Build history of the part. All positions in model axes, mm. Round coordinates to 2 decimals unless told otherwise and drop trailing zeros. Write each loop counter-clockwise with the first axis right and the second up, starting at its lowest first coordinate (ties: lowest second). Pieces come first, ordered by that corner, then holes. Notation, with made-up numbers: (24.25, 55.5) - (56.25, 55.5) arc R12 cw to (56.25, 72.5) - close; hole circle Ø2 at (12.5, 62). An arc over 180 degrees is marked (long way). Write each question's results on one line, items separated by ' | '.
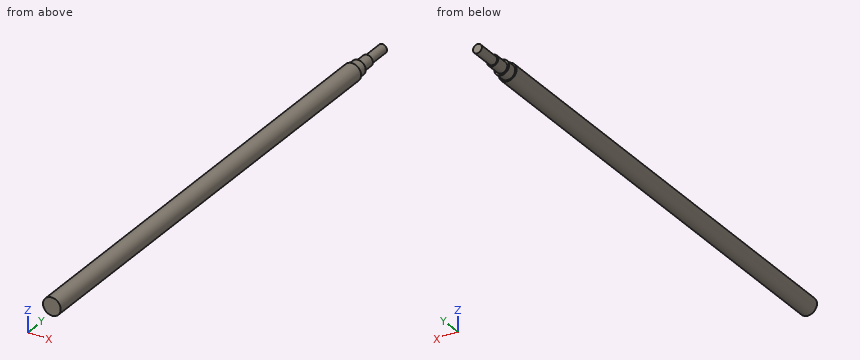
from build123d import *

# Parameters (mm, degrees)
SKETCH1_R           = 9.525
BOSS_EXTRUDE1_DEPTH = 500
SKETCH2_R           = 8
BOSS_EXTRUDE2_DEPTH = 10
SKETCH3_R           = 6
BOSS_EXTRUDE3_DEPTH = 15
SKETCH4_R           = 4.7625
BOSS_EXTRUDE4_DEPTH = 25.4


with BuildPart() as part:
    # Sketch1 → Boss-Extrude1 (new body)
    with BuildSketch(Plane(origin=(0, 0, 0), x_dir=(1, 0, 0), z_dir=(0, 1, 0))):
        with Locations(Location((0, 0, 0), (0, 0, 270))):
            Circle(SKETCH1_R)
    extrude(amount=BOSS_EXTRUDE1_DEPTH)

    # Sketch2 → Boss-Extrude2 (add)
    with BuildSketch(Plane(origin=(0, 500, 0), x_dir=(1, 0, 0), z_dir=(0, 1, 0))):
        with Locations(Location((0, 0, 0), (0, 0, 270))):
            Circle(SKETCH2_R)
    extrude(amount=BOSS_EXTRUDE2_DEPTH)

    # Sketch3 → Boss-Extrude3 (add)
    with BuildSketch(Plane(origin=(0, 510, 0), x_dir=(1, 0, 0), z_dir=(0, 1, 0))):
        with Locations(Location((0, 0, 0), (0, 0, 270))):
            Circle(SKETCH3_R)
    extrude(amount=BOSS_EXTRUDE3_DEPTH)

    # Sketch4 → Boss-Extrude4 (add)
    with BuildSketch(Plane(origin=(0, 525, 0), x_dir=(1, 0, 0), z_dir=(0, 1, 0))):
        with Locations(Location((0, 0, 0), (0, 0, 270))):
            Circle(SKETCH4_R)
    extrude(amount=BOSS_EXTRUDE4_DEPTH)


solid = part.part
(1) Slice it at B-B, the plane x = 0. Write the cut outline in (y, z) (1 decimal).
Worked answers:
outline: (0, -9.5) - (500, -9.5) - (500, -8) - (510, -8) - (510, -6) - (525, -6) - (525, -4.8) - (550.4, -4.8) - (550.4, 4.8) - (525, 4.8) - (525, 6) - (510, 6) - (510, 8) - (500, 8) - (500, 9.5) - (0, 9.5) - close
(2) Flat gauge pins, fed straight in: pin 1 Ø5 at (x, y) = (5, 279) entering from +Z; pin 2 Ø1.5 at (y, z) = (168, 1) entering from -X; pin 3 Ø3 at (x, y) = (-6, 219.5) entering from +Z (3 decimals). Where does each tip first touch, or does it go through?
Worked answers:
pin 1: stops at z = 9.19 | pin 2: stops at x = -9.52 | pin 3: stops at z = 8.395
(3) Slice it at C-C, the plane y = 183. Write the cut outline in (x, z) (3 decimals), and give its area (3 significant figures).
Worked answers:
outline: circle Ø19.05 at (0, 0) | area: 285 mm2
(4) Drill centre lines: probe 1 along Y at (x, z) = (1.5, 6); probe 2 along X at (y, z) = (47, -0.75); probe 3 along Y at (x, z) = (5.25, 7.5). Where is each one in solid material? Low to high. Write a range as [from, to].
Worked answers:
probe 1: y = [0, 510] | probe 2: x = [-9.5, 9.5] | probe 3: y = [0, 500]
(5) Slice it at A-A, the plane z = 0. Write the cut outline in (x, y) (1 decimal).
Worked answers:
outline: (-9.5, 0) - (9.5, 0) - (9.5, 500) - (8, 500) - (8, 510) - (6, 510) - (6, 525) - (4.8, 525) - (4.8, 550.4) - (-4.8, 550.4) - (-4.8, 525) - (-6, 525) - (-6, 510) - (-8, 510) - (-8, 500) - (-9.5, 500) - close
